Solid Edge part; units mm, degrees
sketch "Sketch1" plane through (0, 0, 0) normal (0, 0, 1) x (1, 0, 0)
  circle A0 centre (0, 0) radius 1.5
extrude "Protrusion1" add sketch "Sketch1" along normal blind 6
sketch "Sketch2" plane through (0, 0, 6) normal (0, 0, 1) x (1, 0, 0)
  circle A0 centre (0, 0) radius 2.25
extrude "ProtrusiónExtruida_2" add sketch "Sketch2" along normal blind 1.5
sketch "Sketch3" plane through (0, 0, 7.5) normal (0, 0, 1) x (1, 0, 0)
  line L0 (0, 1.402) -> (1.2141, 0.701)
  line L1 (1.2141, 0.701) -> (1.2141, -0.701)
  line L2 (1.2141, -0.701) -> (0, -1.402)
  line L3 (0, -1.402) -> (-1.2141, -0.701)
  line L4 (-1.2141, -0.701) -> (-1.2141, 0.701)
  line L5 (-1.2141, 0.701) -> (0, 1.402)
extrude "VaciadoExtruido_1" cut sketch "Sketch3" against normal blind 1
chamfer "Chaflán_1" distance 0.4 angle 45 1 edges at (-1.5, 0, 0)
properties material "Acero inoxidable, 303"
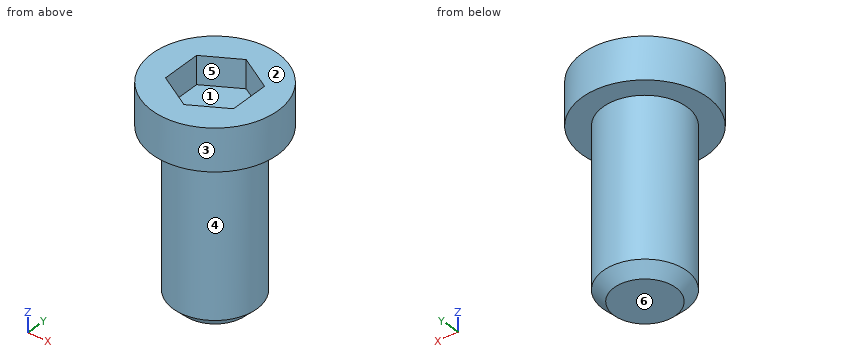
Could you check a few things on this model? Use its own coordinates, in mm. Face numbers are marked on the shaded views. A direction names the side the tool comes from. Coordinates: 2 decimals unless noted, no trailing zeros. Order: outer loops, then holes, each group sorted by start corner. A loop starts at its lowest first (then second) coordinate and runs counter-clockwise, first axis right, second up. Notation, with made-up numbers: (8.25, 80) - (41.25, 80) arc R13 ccw to (41.25, 95) - close; hole circle Ø9 at (39, 30.25). An arc over 180 degrees is marked (long way). Answer in a Markdown table with one row per item. Add a question column.
(1) If we section it at A-A, the plane y = 0: Please give me the cut outline in (x, z), then the cut area to 3 significant figures.
(2) If we section it at D-D, the plane x = 1.6: Please give me the cut outline in (y, z).
(3) If we section it at B-B, the plane z = 7.25: Please give me the cut outline in (x, y).
(4) On a 3-axis mill with a long thin cutter (end or side, diameter ignored), from which of +Z, -Z, +X, -X, +Y, -Y can I reach the whole of each face in a straight line? I mean the marked faces 4, 5 and 6. Say none if no direction works.
(5) If we section it at C-C, the plane z = 5.75: Please give me the cut outline in (x, y), then the cut area to 3 significant figures.
(6) I need wall thicknesses on L1, parallel to Z at x = -0.2, y = -0.6; L2, parallel to Z at x = 1.3, y = 1.25; L3, parallel to X at y = -1.3, z = 7.25. Which ranges of each line are inside material? Lowest first, please.
(7) Will this pin go through, and if not, where does the flat tip stop? pin 1 (0.5 mm diameter, centred on y = 0.5, z = 7, fed in from +X).
(8) If we mould it in two halves opening along Y, with no side actions, what happens to the marked faces 1, 2 and 3? For each: released by +Y, released by -Y, zero draft, split by the parting line, or undercut.
Results are:
| question | item | result |
|---|---|---|
| 1 | outline | (-2.25, 6) - (-1.5, 6) - (-1.5, 0.4) - (-1.1, 0) - (1.1, 0) - (1.5, 0.4) - (1.5, 6) - (2.25, 6) - (2.25, 7.5) - (1.21, 7.5) - (1.21, 6.5) - (-1.21, 6.5) - (-1.21, 7.5) - (-2.25, 7.5) - close |
| 1 | area | 22.2 mm2 |
| 2 | outline | (-1.58, 6) - (1.58, 6) - (1.58, 7.5) - (-1.58, 7.5) - close |
| 3 | outline | circle Ø4.5 at (0, 0); hole (-1.21, -0.7) - (0, -1.4) - (1.21, -0.7) - (1.21, 0.7) - (0, 1.4) - (-1.21, 0.7) - close |
| 4 | face 4 | -Z |
| 4 | face 5 | +Z |
| 4 | face 6 | -Z, +X, -X, +Y, -Y |
| 5 | outline | circle Ø3 at (0, 0) |
| 5 | area | 7.07 mm2 |
| 6 | L1 | z = 0 to 6.5 |
| 6 | L2 | z = 6 to 7.5 |
| 6 | L3 | x = -1.84 to -0.18, 0.18 to 1.84 |
| 7 | pin 1 | stops at x = 2.24 |
| 8 | face 1 | undercut |
| 8 | face 2 | zero draft |
| 8 | face 3 | split by the parting line |
